Can you work these out from the drawing? Everything is in mm from the part's minimum corner. Round coordinates to 2 decimals unless told otherwise and drop trailing zeros. Write each loop counter-clockwise with the first axis right and the second up, starting at its lowest first coordinate (ties: lowest second). Pieces come first, ordered by that corner, then holes. Notation, with made-up numbers: M 45,-5.5 L 51,-5.5 A23 ccw 51,18.5 Z; hole C -5,67 d6. An arc over 180 degrees is marked long. Answer in a Markdown table with one row per item. Add a question column.
(1) I'm going to push flat-ended pins straight in: pin 1 (1 mm diameter, centred on y = 5.5, z = 100, fed in from -X); pin 2 (1.5 mm diameter, centred on x = 26, y = 10, fed in from -Z); pin 3 (5 mm diameter, centred on x = 35.5, y = 9, fed in from -Z). Where does each tip first touch, or does it pass through?
(2) If I drill on probe 1 along Z at (x, y) = (20, 14.5); probe 2 along X at (y, z) = (8, 20); probe 3 along Z at (x, y) = (14, 3.5), over which ranges is the centre line in solid material (lowest first)?
(3) Suppose I cut it at B-B, the plane y = 15.25. Write out the boundary of the cut face in (x, z).
(4) If we mould it in two halves opening along Z, with no side actions, what happens to the marked faces 1, 2 and 3? For each: released by +Z, released by -Z, zero draft, split by the parting line, or undercut.
(5) Suppose I cut it at A-A, the plane x = 20. Write out the boundary of the cut face in (y, z), then the cut area to 3 significant figures.
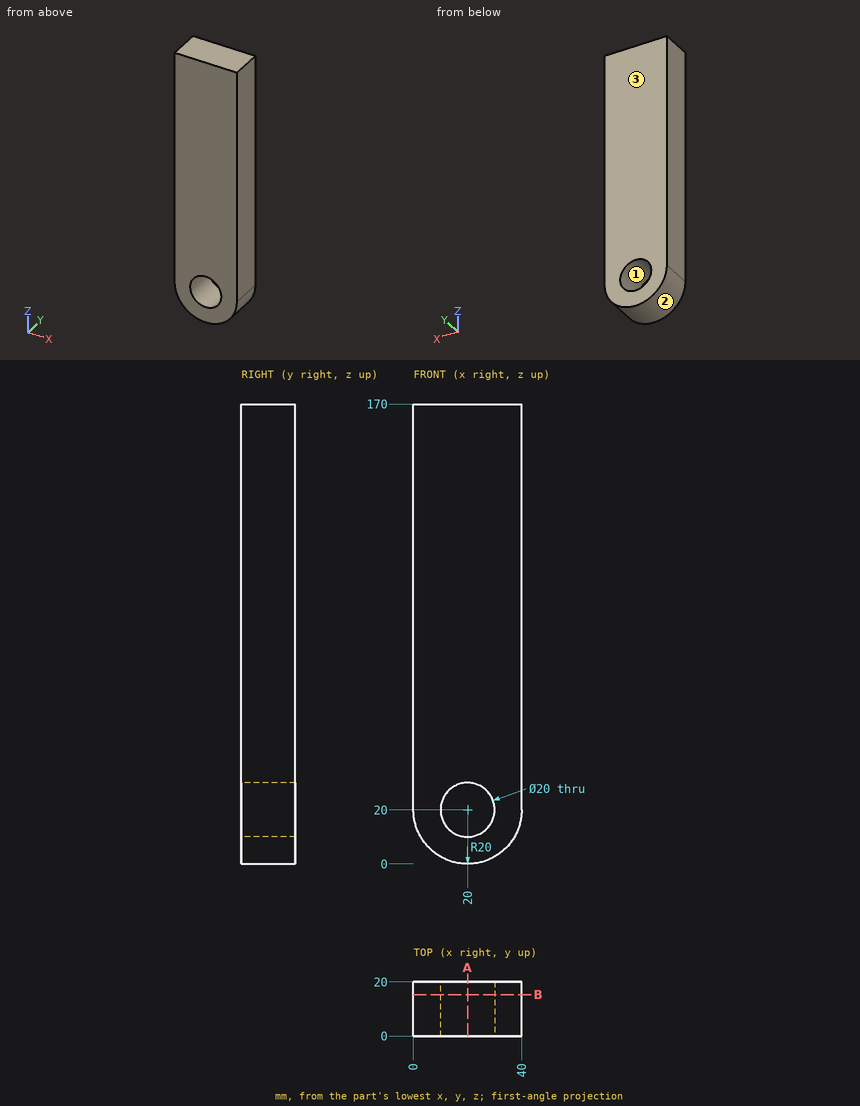
Calculated:
| question | item | result |
|---|---|---|
| 1 | pin 1 | x = 0 |
| 1 | pin 2 | z = 0.7 |
| 1 | pin 3 | z = 4.8 |
| 2 | probe 1 | 0 to 10, 30 to 170 |
| 2 | probe 2 | 0 to 10, 30 to 40 |
| 2 | probe 3 | 0.92 to 12, 28 to 170 |
| 3 | outline | M 0,20 A20 ccw 40,20 L 40,170 L 0,170 Z; hole C 20,20 d20 |
| 4 | face 1 | undercut |
| 4 | face 2 | released by -Z |
| 4 | face 3 | zero draft |
| 5 | outline | M 0,0 L 20,0 L 20,10 L 0,10 Z; M 0,30 L 20,30 L 20,170 L 0,170 Z |
| 5 | area | 3,000 mm² |
